from build123d import *

# Parameters (mm, degrees)
F1_DEPTH = 63.5
F2_DEPTH = 25.4
F3_DEPTH = 7.9375
F5_R     = 6.35


with BuildPart() as f1:
    # F0 (on Front) → F1 (new body, symmetric)
    with BuildSketch(Plane.XZ):
        Polygon((22.225, 9.525), (-41.275, 9.525), (-41.275, -9.525), (41.275, -9.525), (41.275, 9.525), align=None)
    extrude(amount=F1_DEPTH, both=True)

    # F0 (on Front) → F2 (join, symmetric)
    with BuildSketch(Plane.XZ):
        with BuildLine():
            Line((22.225, 30.3276), (22.225, 9.525))
            Line((22.225, 9.525), (41.275, 9.525))
            Line((41.275, 9.525), (41.275, 30.3276))
            ThreePointArc((41.275, 30.3276), (45.92468, 41.55292), (57.15, 46.2026))
            Line((57.15, 46.2026), (60.325, 46.2026))
            Line((60.325, 46.2026), (60.325, 65.2526))
            Line((60.325, 65.2526), (57.15, 65.2526))
            add(Edge.make_bspline(
                [(52.526729, 64.94524), (54.14604, 65.1073), (55.690988, 65.21074), (57.15, 65.2526)],
                knots=[107.655692, 107.655692, 107.655692, 107.655692, 113.106348, 113.106348, 113.106348, 113.106348], degree=3))
            ThreePointArc((52.526729, 64.94524), (30.870508, 53.330729), (22.225, 30.3276))
        make_face()
        Polygon((85.725, 65.2526), (60.325, 65.2526), (60.325, 46.2026), (85.725, 46.2026), (85.725, 52.8701), align=None)
    extrude(amount=F2_DEPTH, both=True)

    # F0 (on Front) → F3 (join, symmetric)
    with BuildSketch(Plane.XZ):
        with BuildLine():
            add(Edge.make_bspline(
                [(-41.275, 9.525), (-40.448051, 35.67537), (20.543785, 61.74439), (52.526729, 64.94524)],
                knots=[0, 0, 0, 0, 107.655692, 107.655692, 107.655692, 107.655692], degree=3))
            Line((-41.275, 9.525), (22.225, 9.525))
            Line((22.225, 9.525), (22.225, 30.3276))
            ThreePointArc((22.225, 30.3276), (30.870508, 53.330729), (52.526729, 64.94524))
        make_face()
    extrude(amount=F3_DEPTH, both=True)

    # F0 (on Front) → F4 (revolve)
    with BuildSketch(Plane.XZ):
        Polygon((85.725, 67.1576), (85.725, 65.2526), (85.725, 52.8701), (85.725, 46.2026), (85.725, 38.5826), (111.125, 38.5826), (111.125, 44.2976), (111.125, 67.1576), (111.125, 72.8726), (85.725, 72.8726), align=None)
    revolve(axis=Axis((85.725, 0, 60.01385), (0, 0, 1)))

    # F5
    f5_edges = [f1.edges().sort_by_distance(p)[0] for p in [
        (41.275, -63.5, 0),
        (41.275, 63.5, 0),
        (-41.275, 63.5, 0),
        (-41.275, -63.5, 0),
    ]]
    fillet(f5_edges, radius=F5_R)


solid = f1.part
Check sheet for the modelled part. Datum: model origin and axes. Units: mm. A direction names the side the tool comes from. Round coordinates to 2 decimals unless told otherwise and drop trailing zeros. Loops run counter-clockwise (first coordinate to the right, second up) from the corner with the lowest first, then second, coordinate; pieces in that order, holes last.
1. Mould release check, pull along X, two halves, no side actions. Record for faces 5 (the cylindrical face through (109.95, 7.63, 55.97)), 6 (the flat face through (-41.275, -1, 0)), 7 (the cylindrical face through (39.464, 61.59, 0.133)): released by +X, released by -X, zero draft, split by the parting line, or undercut.
2. Scan lines: probe 1 along Z at (x, y) = (30, -4) (3 decimals); probe 2 along Y at (x, z) = (11.5, 14); probe 3 along X at (y, z) = (19, 5) (3 decimals). Record each from-to range of solid material in increasing order.
3. Sectioned sample at B-B on y = 44.5. Record the boundary of the cut face in (x, z) (3 decimals), and give its area (3 significant figures).
4. Set-up check for faces 1 (the flat face through (46, -25.4, 44)), 2 (the flat face through (60, 2, 46.203)), 3 (the cylindrical face through (31.1, -16.79, 53.59)), 4 (the flat face through (41.275, -1, 6)): record each of +Z, -Z, +X, -X, +Y, -Y from which the full face is reachable in a straight line by a thin tool's end or side.
5. Sectioned sample at A-A on z = 6. Record the boundary of the cut face in (x, y) (3 decimals).
6. Gauge pin test, flat ends, axial feed: pin 1 Ø16.5 at (x, z) = (16, 45) entering from +Y; pin 2 Ø5 at (x, z) = (45, 39.5) entering from -Y; pin 3 Ø2 at (x, y) = (77, -1) entering from -Z. Record the tip position at first contact, or that the pin passes through.
Recorded:
1. face 5: undercut
1. face 6: released by -X
1. face 7: released by +X
2. probe 1: z = -9.525 to 60.299
2. probe 2: y = -7.94 to 7.94
2. probe 3: x = -41.275 to 41.275
3. outline: (-41.275, -9.525) - (41.275, -9.525) - (41.275, 9.525) - (-41.275, 9.525) - close
3. area: 1,570 mm2
4. face 1: +Z, +X, -X, -Y
4. face 2: -Z
4. face 3: +Z, -X, -Y
4. face 4: -Z, +X, +Y, -Y
5. outline: (-41.275, -57.15) arc R6.35 ccw to (-34.925, -63.5) - (34.925, -63.5) arc R6.35 ccw to (41.275, -57.15) - (41.275, 57.15) arc R6.35 ccw to (34.925, 63.5) - (-34.925, 63.5) arc R6.35 ccw to (-41.275, 57.15) - close
6. pin 1: stops at y = 7.94
6. pin 2: stops at y = -25.4
6. pin 3: stops at z = 38.58
